```python
from build123d import *

# Parameters (mm, degrees)
SKETCH_1_W          = 75
SKETCH_1_H          = 75
EXTRUDE_1_DEPTH     = 2
M4X0_7_1_D          = 3.3
M4X0_7_1_DEPTH      = 11.5
M4X0_7_1_TIP        = 0.991420021
CUT_EXTRUDE_1_DEPTH = 80


with BuildPart() as part:
    # ｽｹｯﾁ1 → ﾎﾞｽ - 押し出し1 (new body)
    with BuildSketch(Plane.XY):
        Rectangle(SKETCH_1_W, SKETCH_1_H)
    extrude(amount=EXTRUDE_1_DEPTH)

    # M4x0.7 ねじ穴1
    with Locations(Plane(origin=(-29.5, -29.5, 0), x_dir=(-1, 0, 0), z_dir=(0, 0, -1))):
        with Locations((0, 0), (0, 59), (-59, 59), (-59, 0)):
            Hole(M4X0_7_1_D / 2, depth=M4X0_7_1_DEPTH)
            with Locations((0, 0, -(M4X0_7_1_DEPTH + M4X0_7_1_TIP / 2))):  # 118° drill point
                Cone(0, M4X0_7_1_D / 2, M4X0_7_1_TIP, mode=Mode.SUBTRACT)

    # ｽｹｯﾁ5 → ｶｯﾄ - 押し出し1 (cut)
    with BuildSketch(Plane(origin=(0, 0, 0), x_dir=(-1, 0, 0), z_dir=(0, 0, -1))):
        with BuildLine():
            ThreePointArc((21.991020895, -17.491020895), (18.80904038, -18.80904038), (17.491020895, -21.991020895))
            Line((17.491020895, -21.991020895), (21.991020895, -21.991020895))
            Line((21.991020895, -21.991020895), (21.991020895, -17.491020895))
        make_face()
        with BuildLine():
            Line((21.991020895, -21.991020895), (17.491020895, -21.991020895))
            ThreePointArc((17.491020895, -21.991020895), (21.991020895, -26.491020895), (26.491020895, -21.991020895))
            ThreePointArc((26.491020895, -21.991020895), (25.17300141, -18.80904038), (21.991020895, -17.491020895))
            Line((21.991020895, -17.491020895), (21.991020895, -21.991020895))
        make_face()
        with BuildLine():
            ThreePointArc((17.491020895, 21.991020895), (18.80904038, 18.80904038), (21.991020895, 17.491020895))
            Line((21.991020895, 17.491020895), (21.991020895, 21.991020895))
            Line((21.991020895, 21.991020895), (17.491020895, 21.991020895))
        make_face()
        with BuildLine():
            Line((21.991020895, 21.991020895), (21.991020895, 17.491020895))
            ThreePointArc((21.991020895, 17.491020895), (25.17300141, 18.80904038), (26.491020895, 21.991020895))
            ThreePointArc((26.491020895, 21.991020895), (21.991020895, 26.491020895), (17.491020895, 21.991020895))
            Line((17.491020895, 21.991020895), (21.991020895, 21.991020895))
        make_face()
        with BuildLine():
            ThreePointArc((-17.491020895, 21.991020895), (-25.17300141, 25.17300141), (-21.991020895, 17.491020895))
            Line((-21.991020895, 17.491020895), (-21.991020895, 21.991020895))
            Line((-21.991020895, 21.991020895), (-17.491020895, 21.991020895))
        make_face()
        with BuildLine():
            Line((-21.991020895, 21.991020895), (-21.991020895, 17.491020895))
            ThreePointArc((-21.991020895, 17.491020895), (-18.80904038, 18.80904038), (-17.491020895, 21.991020895))
            Line((-17.491020895, 21.991020895), (-21.991020895, 21.991020895))
        make_face()
        with BuildLine():
            Line((-17.491020895, -21.991020895), (-21.991020895, -21.991020895))
            Line((-21.991020895, -21.991020895), (-21.991020895, -17.491020895))
            ThreePointArc((-21.991020895, -17.491020895), (-25.17300141, -25.17300141), (-17.491020895, -21.991020895))
        make_face()
        with BuildLine():
            Line((-21.991020895, -21.991020895), (-18.80904038, -18.80904038))
            ThreePointArc((-18.80904038, -18.80904038), (-20.268945449, -17.833562999), (-21.991020895, -17.491020895))
            Line((-21.991020895, -17.491020895), (-21.991020895, -21.991020895))
        make_face()
        with BuildLine():
            ThreePointArc((-17.491020895, -21.991020895), (-17.833562999, -20.268945449), (-18.80904038, -18.80904038))
            Line((-18.80904038, -18.80904038), (-21.991020895, -21.991020895))
            Line((-21.991020895, -21.991020895), (-17.491020895, -21.991020895))
        make_face()
    extrude(amount=-CUT_EXTRUDE_1_DEPTH, mode=Mode.SUBTRACT)


solid = part.part
```
Input: part model. Units: mm. Frame: model coordinates. Coordinates: 2 decimals unless noted, no trailing zeros. Loops run counter-clockwise (first coordinate to the right, second up) from the corner with the lowest first, then second, coordinate; pieces in that order, holes last. Notation, with made-up numbers: M -4,12 L 47,12 A26 ccw 47,27 Z; hole C 1.25,77.5 d5. An arc over 180 degrees is marked long. Use a Markdown table: item, result. Add a question column.
1) Section C-C, the plane z = 1.6. Give the number of separate pieces and of enclosed holes in the cut face, plus the area to 3 significant figures.
2) Pin query (flat end, axial travel): P1, Ø3, axis at x = -29.5, y = -29.5, coming from the +Z side. Return the tip coordinate at first contact, or that it passes through.
3) Section A-A, the plane y = 29.5. Return the cut outline in (x, z).
4) Draft query along X for faces 1 (the cylindrical face through (29.285, 31.136, 1.014)), 2 (the flat face through (-1, 1, 0)), 3 (the flat face through (37.5, -1, 1)), 4 (the flat face through (-37.5, -1, 1)). Return one class per face: +X half, -X half, draft (parallel to the pull), parting line (faces both ways), or undercut.
5) Line query: L1, parallel to Y at x = 29.5, z = 0.55; L2, parallel to Y at x = -21, z = 1.2; L3, parallel to X at y = -31, z = 0.55. Output: solid intervals per line, ascending. Write a range as from..to.
Answer below:
| question | item | result |
|---|---|---|
| 1 | separate pieces | 1 |
| 1 | enclosed holes | 8 |
| 1 | area | 5,340 mm2 |
| 2 | P1 | through |
| 3 | outline | M -37.5,0 L -31.15,0 L -31.15,2 L -37.5,2 Z; M -27.85,0 L 27.85,0 L 27.85,2 L -27.85,2 Z; M 31.15,0 L 37.5,0 L 37.5,2 L 31.15,2 Z |
| 4 | face 1 | undercut |
| 4 | face 2 | draft |
| 4 | face 3 | +X half |
| 4 | face 4 | -X half |
| 5 | L1 | -37.5..-31.15, -27.85..27.85, 31.15..37.5 |
| 5 | L2 | -37.5..-26.38, -17.6..17.6, 26.38..37.5 |
| 5 | L3 | -37.5..-30.19, -28.81..28.81, 30.19..37.5 |
